from build123d import *

# Parameters (mm, degrees)
F0_W         = 101.6
F0_H         = 101.6
F1_DEPTH     = 101.6
F2_R         = 31.75
F1_FACE1_W   = 101.6
F1_FACE1_H   = 101.6
F3_DEPTH     = 101.6
F4_R         = 31.75
F5_DEPTH     = 101.6
F6_R         = 31.75
F7_DEPTH     = 101.6
F8_R         = 5.08
F9_T1_DEPTH  = 91.44
F9_S5_W      = 5.08
F9_S5_H      = 5.08
F9_T6_DEPTH  = 5.08
F9_S11_W     = 5.08
F9_S11_H     = 5.08
F9_T12_DEPTH = 5.08
F10_SIZE     = 5.08


# Not quite as in the source:
# - a fillet or chamfer that OpenCascade refuses, or shapes differently, is made with other operations: its cross-section is extruded or revolved along the edge and cut away or added


with BuildPart() as f1:
    # F0 (on Top) → F1 (new body)
    with BuildSketch(Plane.XY):
        with Locations((50.8, 50.8)):
            Rectangle(F0_W, F0_H)
    extrude(amount=F1_DEPTH)

    # F2 (on face) + F1_face1 (on face) → F3 (cut)
    with BuildSketch(Plane.YZ.offset(101.6)):
        with Locations((50.8, 50.8)):
            Circle(F2_R)
    with BuildSketch(Plane(origin=(0, 50.8, 50.8), x_dir=(0, -1, 0), z_dir=(-1, 0, 0))):
        Rectangle(F1_FACE1_W, F1_FACE1_H)
    extrude(amount=-F3_DEPTH, dir=(1, 0, 0), mode=Mode.SUBTRACT)

    # F4 (on face) → F5 (cut)
    with BuildSketch(Plane.XZ):
        with Locations((50.8, 50.8)):
            Circle(F4_R)
    extrude(amount=-F5_DEPTH, mode=Mode.SUBTRACT)

    # F6 (on face) → F7 (cut)
    with BuildSketch(Plane(origin=(0, 0, 0), x_dir=(1, 0, 0), z_dir=(0, 0, -1))):
        with Locations((50.8, -50.8)):
            Circle(F6_R)
    extrude(amount=-F7_DEPTH, mode=Mode.SUBTRACT)

    # F8
    f8_edges = [f1.edges().sort_by_distance(p)[0] for p in [
        (50.8, 0, 101.6),
        (101.6, 50.8, 101.6),
        (50.8, 101.6, 101.6),
        (0, 50.8, 101.6),
        (101.6, 101.6, 50.8),
        (101.6, 0, 50.8),
        (101.6, 50.8, 0),
        (50.8, 101.6, 0),
        (0, 101.6, 50.8),
        (50.8, 0, 0),
        (0, 0, 50.8),
    ]]
    fillet(f8_edges, radius=F8_R)

    # F9: fillet of radius 5.08 on 1 edges, made by hand

    # F9_s2 → F9_t1 (cut)
    with BuildSketch(Plane.XZ.offset(-96.52)):
        with BuildLine():
            ThreePointArc((0, 5.08), (1.4878975516, 1.4878975516), (5.08, 0))
            Line((5.08, 0), (0, 0))
            Line((0, 0), (0, 5.08))
        make_face()
    extrude(amount=F9_T1_DEPTH, mode=Mode.SUBTRACT)


with BuildPart() as f9_tool4:
    # F9_s5 → F9_t6 (new body)
    with BuildSketch(Plane.YZ.offset(5.08)):
        with Locations((99.06, 2.54)):
            Rectangle(F9_S5_W, F9_S5_H)
    extrude(amount=-F9_T6_DEPTH)

    # F9_s7 → F9_t8 (revolve, cut)
    with BuildSketch(Plane(origin=(5.08, 96.52, 5.08), x_dir=(0, -0.7071067812, 0.7071067812), z_dir=(0, -0.7071067812, -0.7071067812))):
        with BuildLine():
            ThreePointArc((0, -5.08), (5.08, 0), (0, 5.08))
            Line((0, 5.08), (0, -5.08))
        make_face()
    revolve(axis=Axis((5.08, 96.52, 5.08), (-1, 0, 0)), mode=Mode.SUBTRACT)


with BuildPart() as f1_1:
    add(f1.part)

    # F9_t3: cut F9_tool4
    add(f9_tool4.part, mode=Mode.SUBTRACT)


with BuildPart() as f9_tool10:
    # F9_s11 → F9_t12 (new body)
    with BuildSketch(Plane.YZ.offset(5.08)):
        with Locations((2.54, 2.54)):
            Rectangle(F9_S11_W, F9_S11_H)
    extrude(amount=-F9_T12_DEPTH)

    # F9_s13 → F9_t14 (revolve, cut)
    with BuildSketch(Plane(origin=(5.08, 5.08, 5.08), x_dir=(0, 0.7071067812, 0.7071067812), z_dir=(0, -0.7071067812, 0.7071067812))):
        with BuildLine():
            ThreePointArc((0, -5.08), (5.08, 0), (0, 5.08))
            Line((0, 5.08), (0, -5.08))
        make_face()
    revolve(axis=Axis((5.08, 5.08, 5.08), (-1, 0, 0)), mode=Mode.SUBTRACT)


with BuildPart() as f1_2:
    add(f1_1.part)

    # F9_t9: cut F9_tool10
    add(f9_tool10.part, mode=Mode.SUBTRACT)

    # F10
    f10_edges = [f1_2.edges().sort_by_distance(p)[0] for p in [
        (101.6, 19.05, 50.8),
        (0, 19.05, 50.8),
        (19.05, 50.8, 0),
        (19.05, 0, 50.8),
        (19.05, 50.8, 101.6),
        (19.05, 101.6, 50.8),
    ]]
    chamfer(f10_edges, length=F10_SIZE)


solid = f1_2.part
Could you check a few things on this model? Use its own coordinates, in mm. Round coordinates to 2 decimals unless told otherwise and drop trailing zeros. Write each loop counter-clockwise with the first axis right and the second up, starting at its lowest first coordinate (ties: lowest second). Pieces come first, ordered by that corner, then holes. Notation, with made-up numbers: (52, 45.5) - (75, 45.5) arc R24 ccw to (75, 67.5) - close; hole circle Ø11 at (16, -38.75). An arc over 180 degrees is marked (long way). Put each result on its own line as item: value. Start each with the question number.
(1) Will these pins go through, and if not, where does the flat tip stop? pin 1 (10 mm diameter, centred on x = 58, z = 21.5, fed in from -Y); pin 2 (2 mm diameter, centred on x = 68.5, z = 80.5, fed in from +Y).
(2) I need wall thicknesses on probe 1 along Y at (x, z) = (50.8, 14); probe 2 along Z at (x, y) = (5, 97); probe 3 along Z at (x, y) = (76.5, 91). Which ranges of each line are inside material? Lowest first, please.
(3) Thinking about a two-plate mould opening in Y: for faces 1 (the cylindrical face through (14.29, 19.08, 52.2)), 2 (the cylindrical face through (1.449, 100.072, 51.44)), 3 (the flat face through (30, 82, 101.6)), which applies, released by +Y, released by -Y, zero draft, split by the parting line, or undercut?
(4) I want a section at D-D, the plane z = 24.5. Give the number of separate pieces and of enclosed holes in the cut face, plus the area to 3 significant figures.
(5) I want a section at A-A, the plane z = 50.8. Please give me the cut outline in (x, y), plus the area to 3 significant figures.
(6) I want a section at C-C, the plane z = 12. Please give me the cut outline in (x, y).
Here are the results:
1. pin 1: stops at y = 1.66
1. pin 2: stops at y = 100.34
2. probe 1: y = 0.03 to 19.05, 82.55 to 101.57
2. probe 2: z = 0.02 to 101.58
2. probe 3: z = 0 to 32.16, 69.44 to 101.6
3. face 1: undercut
3. face 2: released by +Y
3. face 3: zero draft
4. separate pieces: 4
4. enclosed holes: 0
4. area: 4,010 mm^2
5. outline: (0, 5.08) arc R5.08 ccw to (5.08, 0) - (13.97, 0) - (19.05, 5.08) - (19.05, 19.05) - (5.08, 19.05) - (0, 13.97) - close; (0, 87.63) - (5.08, 82.55) - (19.05, 82.55) - (19.05, 96.52) - (13.97, 101.6) - (5.08, 101.6) arc R5.08 ccw to (0, 96.52) - close; (82.55, 5.08) - (87.63, 0) - (96.52, 0) arc R5.08 ccw to (101.6, 5.08) - (101.6, 13.97) - (96.52, 19.05) - (82.55, 19.05) - close; (82.55, 82.55) - (96.52, 82.55) - (101.6, 87.63) - (101.6, 96.52) arc R5.08 ccw to (96.52, 101.6) - (87.63, 101.6) - (82.55, 96.52) - close
5. area: 1,330 mm^2
6. outline: (0, 5.08) arc R5.08 ccw to (5.08, 0) - (96.52, 0) arc R5.08 ccw to (101.6, 5.08) - (101.6, 96.52) arc R5.08 ccw to (96.52, 101.6) - (5.08, 101.6) arc R5.08 ccw to (0, 96.52) - close; hole circle Ø63.5 at (50.8, 50.8)
